from build123d import *

# Parameters (mm, degrees)
F0_W     = 76.2
F0_H     = 38.1
F1_DEPTH = 2.032
F2_W     = 76.2
F2_H     = 38.1
F2_W_2   = 72.136
F2_H_2   = 34.036
F3_DEPTH = 12.7
F4_R     = 1.27
F5_DEPTH = 2.54
F6_W     = 16.51
F6_H     = 5.08
F6_W_2   = 25.4
F7_DEPTH = 2.032
F8_R     = 5.08
F9_R     = 5.08


with BuildPart() as f1:
    # F0 (on Top) → F1 (new body)
    with BuildSketch(Plane.XY):
        Rectangle(F0_W, F0_H)
    extrude(amount=F1_DEPTH)

    # F2 (on face) → F3 (join)
    with BuildSketch(Plane.XY.offset(2.032)):
        Rectangle(F2_W, F2_H)
        Rectangle(F2_W_2, F2_H_2, mode=Mode.SUBTRACT)
    extrude(amount=F3_DEPTH)

    # F4 (on face) → F5 (join)
    with BuildSketch(Plane.XY.offset(2.032)):
        with Locations((-28.575, 11.43)):
            Circle(F4_R)
        with Locations((-28.575, -11.43)):
            Circle(F4_R)
        with Locations((28.575, -11.43)):
            Circle(F4_R)
        with Locations((28.575, 11.43)):
            Circle(F4_R)
    extrude(amount=F5_DEPTH)

    # F6 (on face) → F7 (cut)
    with BuildSketch(Plane.XZ.offset(19.05)):
        with Locations((-20.32, 4.572)):
            Rectangle(F6_W, F6_H)
        with Locations((15.875, 4.572)):
            Rectangle(F6_W_2, F6_H)
    extrude(amount=-F7_DEPTH, mode=Mode.SUBTRACT)

    # F8
    f8_edges = [f1.edges().sort_by_distance(p)[0] for p in [
        (-36.068, 17.018, 8.382),
        (-36.068, -17.018, 8.382),
        (36.068, 17.018, 8.382),
        (36.068, -17.018, 8.382),
    ]]
    fillet(f8_edges, radius=F8_R)

    # F9
    f9_edges = [f1.edges().sort_by_distance(p)[0] for p in [
        (-38.1, -19.05, 7.366),
        (38.1, -19.05, 7.366),
        (38.1, 19.05, 7.366),
        (-38.1, 19.05, 7.366),
    ]]
    fillet(f9_edges, radius=F9_R)


solid = f1.part
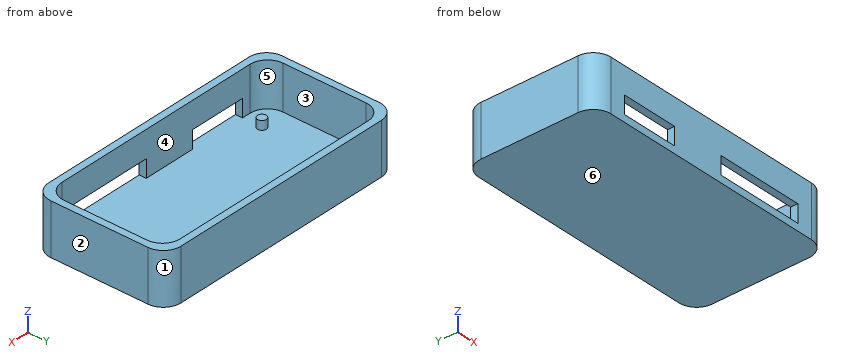
Work out the finished part from the listing and answer in its coordinate system (mm). Face numbers are marked on the shaded views. A direction names the side the tool comes from. Coordinates: 2 decimals unless noted, no trailing zeros. Order: outer loops, then holes, each group sorted by start corner. A loop starts at its lowest first (then second) coordinate and runs counter-clockwise, first axis right, second up. Notation, with made-up numbers: (57.25, 64.25) - (114.25, 64.25) arc R22 cw to (114.25, 77.25) - close; hole circle Ø11 at (52.25, -26). An arc over 180 degrees is marked (long way). Put each result on its own line as item: value. Start each with the question number.
1) Find section B-B (x = -17.5). Give the vertices of the cut face in (y, z), plus the area to 3 significant figures.
2) Find the intervals of material crossed by line 1 (X direction, y = 8, z = 14); line 2 (Y direction, x = -12, z = 3.5); line 3 (Y direction, x = -27.5, z = 3.75), in increasing order. Write a range as from..to.
3) Find section C-C (y = -6). Give the vertices of the cut face in (x, z).
4) For a pull along Y with two mould halves and no side action, classify the marked faces 1, 2, 3 and 4 as released by +Y, released by -Y, zero draft, split by the parting line, or undercut.
5) Find section D-D (x = -8). Give the vertices of the cut face in (y, z).
6) For the marked faces 5 and 6, determine the directions among +Z, -Z, +X, -X, +Y, -Y from which every point of the face is accessible in a straight line to the end or side of a thin tool.
7) Flat-ended cylindrical pins translate along their axes: pin 1 (1.6 mm diameter, centred on y = -18, z = 5.5, fed in from -X); pin 2 (0.6 mm diameter, centred on y = -18, z = 3.5, fed in from -X); pin 3 (2 mm diameter, centred on x = -29, y = -11, fed in from +Z). Find the tip coordinate at first contact, or state that the pin passes through.
8) Find section A-A (z = 9). Give the vertices of the cut face in (x, y), plus the area to 3 significant figures.
Results list:
1. outline: (-19.05, 0) - (19.05, 0) - (19.05, 14.73) - (17.02, 14.73) - (17.02, 2.03) - (-19.05, 2.03) - close; (-19.05, 7.11) - (-17.02, 7.11) - (-17.02, 14.73) - (-19.05, 14.73) - close
1. area: 119 mm^2
2. line 1: x = -38.1..-36.07, 36.07..38.1
2. line 2: y = -19.05..-17.02, 17.02..19.05
2. line 3: y = -12.11..-10.75, 10.75..12.11, 17.02..19.05
3. outline: (-38.1, 0) - (38.1, 0) - (38.1, 14.73) - (36.07, 14.73) - (36.07, 2.03) - (-36.07, 2.03) - (-36.07, 14.73) - (-38.1, 14.73) - close
4. face 1: released by +Y
4. face 2: zero draft
4. face 3: undercut
4. face 4: undercut
5. outline: (-19.05, 0) - (19.05, 0) - (19.05, 14.73) - (17.02, 14.73) - (17.02, 2.03) - (-17.02, 2.03) - (-17.02, 14.73) - (-19.05, 14.73) - close
6. face 5: +Z
6. face 6: -Z, +X, -X, +Y, -Y
7. pin 1: stops at x = -36.94
7. pin 2: stops at x = -36.47
7. pin 3: stops at z = 4.57
8. outline: (-38.1, -13.97) arc R5.08 ccw to (-33.02, -19.05) - (33.02, -19.05) arc R5.08 ccw to (38.1, -13.97) - (38.1, 13.97) arc R5.08 ccw to (33.02, 19.05) - (-33.02, 19.05) arc R5.08 ccw to (-38.1, 13.97) - close; hole (-36.07, -11.94) arc R5.08 ccw to (-30.99, -17.02) - (30.99, -17.02) arc R5.08 ccw to (36.07, -11.94) - (36.07, 11.94) arc R5.08 ccw to (30.99, 17.02) - (-30.99, 17.02) arc R5.08 ccw to (-36.07, 11.94) - close
8. area: 448 mm^2
